```python
from build123d import *

# Parameters (mm, degrees)
F0_R     = 1.5
F1_DEPTH = 1.5


with BuildPart() as f1:
    # F0 (on Top) → F1 (new body)
    with BuildSketch(Plane.XY):
        Polygon((0, 39.600004), (-23.670001, 39.600004), (-23.670001, 14.86), (-23.670001, 13.36), (-23.670001, 9.36), (0, 9.36), align=None)
        with Locations((-21.170001, 14.86)):
            Circle(F0_R, mode=Mode.SUBTRACT)
        with Locations((-2.5, 14.86)):
            Circle(F0_R, mode=Mode.SUBTRACT)
        with Locations((-21.170001, 29.448288)):
            Circle(F0_R, mode=Mode.SUBTRACT)
        with Locations((-2.5, 29.448288)):
            Circle(F0_R, mode=Mode.SUBTRACT)
    extrude(amount=F1_DEPTH)


solid = f1.part
```
Part model, mm, in its own coordinate system. Coordinates: 2 decimals unless noted, no trailing zeros. Write each loop counter-clockwise with the first axis right and the second up, starting at its lowest first coordinate (ties: lowest second). Pieces come first, ordered by that corner, then holes.
Item 1: Slice it at B-B (y = 14.86). Write the cut outline in (x, z).
Item 2: Probe line 1 (Y direction, x = -2.5, z = 0.8); line 2 (X direction, y = 14.5, z = 1.35); line 3 (X direction, y = 13.5, z = 1). List the from-to ranges inside material, lowest first.
Item 3: Pin check, flat tip, straight feed: pin 1 (2.5 mm diameter, centred on x = -2.5, y = 29.45, fed in from +Z). Stop position of the tip, or through.
Item 4: Slice it at A-A (x = -2.5). Write the cut outline in (y, z), and give its area (3 significant figures).
Item 5: Mould opens along X. For faces 1 (the face through (-2.695, 16.347, 0.74)), 2 (the face through (-22.67, 14.93, 0.74)), 3 (the face through (-12, 25, 0)), 4 (the face through (0, 24, 1)) say: released by +X, released by -X, zero draft, split by the parting line, or undercut.
Item 6: Slice it at C-C (z = 1.2). Write the cut outline in (x, y), and give its area (3 significant figures).
Results found:
1. outline: (-23.67, 0) - (-22.67, 0) - (-22.67, 1.5) - (-23.67, 1.5) - close; (-19.67, 0) - (-4, 0) - (-4, 1.5) - (-19.67, 1.5) - close; (-1, 0) - (0, 0) - (0, 1.5) - (-1, 1.5) - close
2. line 1: y = 9.36 to 13.36, 16.36 to 27.95, 30.95 to 39.6
2. line 2: x = -23.67 to -22.63, -19.71 to -3.96, -1.04 to 0
2. line 3: x = -23.67 to -21.8, -20.54 to -3.13, -1.87 to 0
3. pin 1: passes through
4. outline: (9.36, 0) - (13.36, 0) - (13.36, 1.5) - (9.36, 1.5) - close; (16.36, 0) - (27.95, 0) - (27.95, 1.5) - (16.36, 1.5) - close; (30.95, 0) - (39.6, 0) - (39.6, 1.5) - (30.95, 1.5) - close
4. area: 36.4 mm2
5. face 1: undercut
5. face 2: undercut
5. face 3: zero draft
5. face 4: released by +X
6. outline: (-23.67, 9.36) - (0, 9.36) - (0, 39.6) - (-23.67, 39.6) - close; hole circle Ø3 at (-21.17, 14.86); hole circle Ø3 at (-21.17, 29.45); hole circle Ø3 at (-2.5, 14.86); hole circle Ø3 at (-2.5, 29.45)
6. area: 688 mm2
